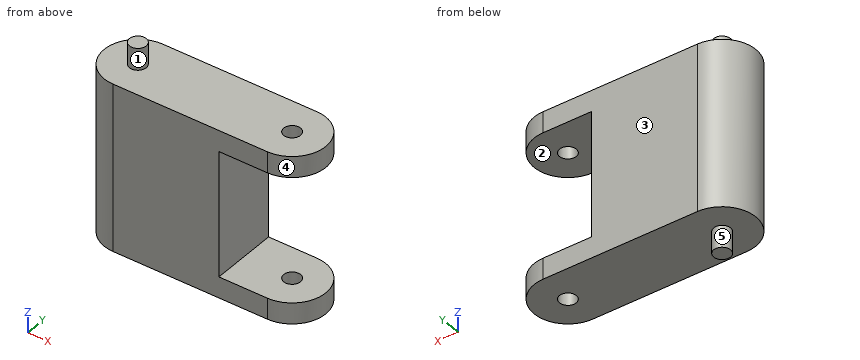
from build123d import *

# Parameters (mm, degrees)
SALIENTE_EXTRUIR1_DEPTH      = 199
CROQUIS6_R                   = 9.988
CORTAR_EXTRUIR3_DEPTH        = 240
SALIENTE_EXTRUIR3_DEPTH      = 26
SALIENTE_EXTRUIR3_DEPTH_BACK = 225
CROQUIS3_R                   = 10
CROQUIS12_W                  = 123.646893132
CROQUIS12_H                  = 149
CORTAR_EXTRUIR7_DEPTH        = 122


with BuildPart() as part:
    # Croquis2 → Saliente-Extruir1 (new body)
    with BuildSketch(Plane.XY):
        with BuildLine():
            Line((0, 40), (183.351967946, 40))
            ThreePointArc((183.351967946, 40), (223.351967946, 0), (183.351967946, -40))
            Line((183.351967946, -40), (0, -40))
            ThreePointArc((0, -40), (-40, 0), (0, 40))
        make_face()
    extrude(amount=SALIENTE_EXTRUIR1_DEPTH)

    # Croquis6 → Cortar-Extruir3 (cut)
    with BuildSketch(Plane(origin=(0, 0, 0), x_dir=(-1, 0, 0), z_dir=(0, 0, -1))):
        with Locations((-183.351967946, 0)):
            Circle(CROQUIS6_R)
    extrude(amount=-CORTAR_EXTRUIR3_DEPTH, mode=Mode.SUBTRACT)

    # Croquis3 → Saliente-Extruir3 (add, two sides: drawn at the far end of the back side and taken through both)
    with BuildSketch(Plane.XY.offset(199).offset(-SALIENTE_EXTRUIR3_DEPTH_BACK)):
        Circle(CROQUIS3_R)
    extrude(amount=SALIENTE_EXTRUIR3_DEPTH + SALIENTE_EXTRUIR3_DEPTH_BACK)

    # Croquis12 → Cortar-Extruir7 (cut)
    with BuildSketch(Plane(origin=(0, 40, 0), x_dir=(1, 0, 0), z_dir=(0, 1, 0))):
        with Locations((187.658688953, -99.5)):
            Rectangle(CROQUIS12_W, CROQUIS12_H)
    extrude(amount=-CORTAR_EXTRUIR7_DEPTH, mode=Mode.SUBTRACT)


solid = part.part
Design review of the part built by this model. Coordinates are the model's own, in mm. Face numbers are marked on the shaded views. A direction names the side the tool comes from. Give positions to 0.01 mm unless a question says otherwise; leave off trailing zeros. Loops run counter-clockwise (first coordinate to the right, second up) from the corner with the lowest first, then second, coordinate; pieces in that order, holes last. Notation, with made-up numbers: (-18, 34.5) - (25, 34.5) arc R14 cw to (25, 52.5) - close; hole circle Ø4 at (47.5, 36). An arc over 180 degrees is marked (long way). Use CSV: the item, a comma, the result in double quotes. Start each with the question number.
1. Add section A-A (y = 0). State the section outline as (x, z) points, plus the area to 3 significant figures.
2. Add section B-B (x = -6.5). State the section outline as (y, z) points.
3. Add section D-D (y = 16). State the section outline as (x, z) points, plus the area to 3 significant figures.
4. Wall thickness on L1, parallel to Z at x = 143.5, y = -14; L2, parallel to Z at x = 79, y = 10; L3, parallel to X at y = -6.5, z = 11: over which ranges is each line inside the solid? List them lowest first.
5. Machinability: for the marked faces 1, 2, 3, 4 and 5, which of the approach directions +Z, -Z, +X, -X, +Y, -Y give a long, thin tool a straight path to every point of the face, cutting with its end or side? Answer none if there is none.
6. Insertion check: P1, Ø2, axis at y = -30.5, z = 101, coming from the +X side; P2, Ø23, axis at x = 183.35, y = 0, coming from the +Z side; P3, Ø5, axis at x = 146.5, y = -7, coming from the -Z side. Each pin has a flat end and moves straight along its axis. Give the tip position at first contact, or say it passes through.
7. Add section C-C (z = 45). State the section outline as (x, y) points, plus the area to 3 significant figures.
Results found:
1,outline,"(-40, 0) - (-10, 0) - (-10, -26) - (10, -26) - (10, 0) - (173.36, 0) - (173.36, 25) - (125.84, 25) - (125.84, 174) - (173.36, 174) - (173.36, 199) - (10, 199) - (10, 225) - (-10, 225) - (-10, 199) - (-40, 199) - close; (193.34, 0) - (223.35, 0) - (223.35, 25) - (193.34, 25) - close; (193.34, 174) - (223.35, 174) - (223.35, 199) - (193.34, 199) - close"
1,area,"37,900 mm²"
2,outline,"(-39.47, 0) - (-7.6, 0) - (-7.6, -26) - (7.6, -26) - (7.6, 0) - (39.47, 0) - (39.47, 199) - (7.6, 199) - (7.6, 225) - (-7.6, 225) - (-7.6, 199) - (-39.47, 199) - close"
3,outline,"(-36.66, 0) - (220.01, 0) - (220.01, 25) - (125.84, 25) - (125.84, 174) - (220.01, 174) - (220.01, 199) - (-36.66, 199) - close"
3,area,"37,000 mm²"
4,L1,"z = 0 to 25, 174 to 199"
4,L2,"z = 0 to 199"
4,L3,"x = -39.47 to 175.77, 190.94 to 222.82"
5,face 1,"+Z"
5,face 2,"+X, +Y, -Y"
5,face 3,"+Z, -Z, +X, -X, +Y"
5,face 4,"+Z, -Z, +X"
5,face 5,"-Z"
6,P1,"stops at x = 125.84"
6,P2,"stops at z = 199"
6,P3,"stops at z = 0"
7,outline,"(0, -40) - (125.84, -40) - (125.84, 40) - (0, 40) arc R40 ccw to start"
7,area,"12,600 mm²"
